Check sheet for the modelled part. Datum: model origin and axes. Units: mm. Face numbers are marked on the shaded views. A direction names the side the tool comes from. Coordinates: 2 decimals unless noted, no trailing zeros. Loops run counter-clockwise (first coordinate to the right, second up) from the corner with the lowest first, then second, coordinate; pieces in that order, holes last. Notation, with made-up numbers: (-38, -17.5) - (-12, -17.5) arc R32 cw to (-12, 13.5) - close; hole circle Ø2 at (67, 88.25). An arc over 180 degrees is marked (long way). Use a Markdown table: item, result. Add a question column.
1) Draft check along X on the marked faces 4, 5, 6 and 7. Enter one of: pulls with the +X half, pulls with the -X half, needs draft (parallel to the pull), parting line crosses it, or undercut.
2) Sectioned sample at D-D, the plane x = -8.5. Enter the section's corners in (y, z), then the cut area to 3 significant figures.
3) Sectioned sample at B-B, the plane y = -46. Enter the section's corners in (x, z), then the cut area to 3 significant figures.
4) Tool access check on the marked faces 1, 2 and 3. Record the directions out of +Z, -Z, +X, -X, +Y, -Y that give a thin tool (end or side, any length) a straight path to the whole face; none if there is none.
5) Go/stop test with flat-tipped pins: P1, Ø8, axis at y = -9, z = 138.5, coming from the +X side; P2, Ø9, axis at x = -8.5, z = 137.15, coming from the +Y side; P3, Ø2.5, axis at x = 14.5, y = -43.5, coming from the +Z side; P4, Ø6, axis at x = -1.5, z = 132.5, coming from the -Y side. Record where each tip stops, or that it passes through.
6) Sectioned sample at A-A, the plane x = 0. Enter the section's corners in (y, z).
7) Sectioned sample at C-C, the plane y = 1.5. Enter the section's corners in (x, z).
8) Thickness scan on line 1 (X direction, y = -3.2, z = 137.15); line 2 (Y direction, x = -17, z = 124); line 3 (Y direction, x = -9, z = 139). Record the ranges inside material, lowest first.
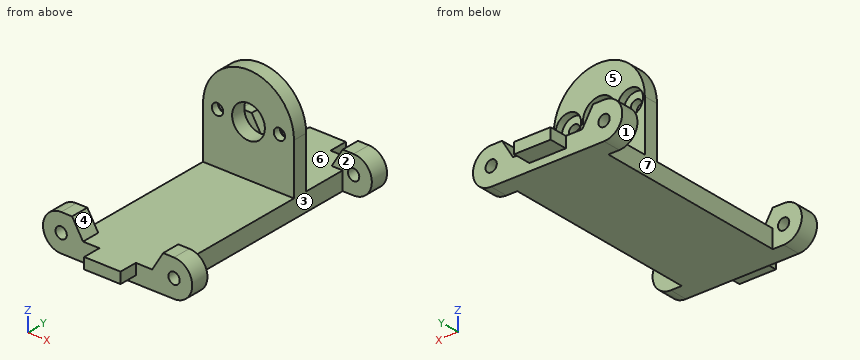
from build123d import *

# Parameters (mm, degrees)
SKETCH11_R          = 1.55
SKETCH11_R_2        = 4.5
BOSS_EXTRUDE1_DEPTH = 4
BOSS_EXTRUDE2_DEPTH = 5
SKETCH13_R          = 3.5
CUT_EXTRUDE1_DEPTH  = 2
SKETCH14_R          = 1.55
BOSS_EXTRUDE3_DEPTH = 5
BOSS_EXTRUDE4_START = -5
SKETCH15_R          = 1.55
BOSS_EXTRUDE4_DEPTH = 5
SKETCH16_W          = 10
SKETCH16_H          = 3
BOSS_EXTRUDE5_DEPTH = 5
SKETCH17_W          = 10
SKETCH17_H          = 3
BOSS_EXTRUDE6_DEPTH = 5


with BuildPart() as part:
    # Sketch11 → Boss-Extrude1 (new body)
    with BuildSketch(Plane(origin=(0, 0, 51.65), x_dir=(1, 0, 0), z_dir=(0, -1, 0))):
        with BuildLine():
            Line((12.5, 85.5), (12.5, 71.5))
            Line((12.5, 71.5), (-12.5, 71.5))
            Line((-12.5, 71.5), (-12.5, 85.5))
            ThreePointArc((-12.5, 85.5), (0, 98), (12.5, 85.5))
        make_face()
        with Locations(Location((-8.5, 85.5, 0), (0, 0, 270))):
            Circle(SKETCH11_R, mode=Mode.SUBTRACT)
        with Locations(Location((8.5, 85.5, 0), (0, 0, 270))):
            Circle(SKETCH11_R, mode=Mode.SUBTRACT)
        with Locations(Location((0, 85.5, 0), (0, 0, 270))):
            Circle(SKETCH11_R_2, mode=Mode.SUBTRACT)
    extrude(amount=BOSS_EXTRUDE1_DEPTH)

    # Sketch12 → Boss-Extrude2 (add)
    with BuildSketch(Plane(origin=(0, 0, 123.15), x_dir=(-1, 0, 0), z_dir=(0, 0, -1))):
        Polygon((-12.5, 0), (-12.5, 17), (12.5, 17), (12.5, 0), (12.5, -4), (12.5, -47), (-12.5, -47), (-12.5, -4), align=None)
    extrude(amount=BOSS_EXTRUDE2_DEPTH)

    # Sketch13 → Cut-Extrude1 (cut)
    with BuildSketch(Plane(origin=(0, 0, 0), x_dir=(1, 0, 0), z_dir=(0, 1, 0))):
        with Locations(Location((-8.5, -137.15, 0), (0, 0, 270))):
            Circle(SKETCH13_R)
        with Locations(Location((8.5, -137.15, 0), (0, 0, 270))):
            Circle(SKETCH13_R)
    extrude(amount=-CUT_EXTRUDE1_DEPTH, mode=Mode.SUBTRACT)

    # Sketch14 → Boss-Extrude3 (add)
    with BuildSketch(Plane(origin=(0, 17, 0), x_dir=(1, 0, 0), z_dir=(0, 1, 0))):
        with BuildLine():
            Line((15.5, -118.15), (-15.5, -118.15))
            ThreePointArc((-15.5, -118.15), (-20.5, -123.15), (-15.5, -128.15))
            Line((-15.5, -128.15), (-12.5, -128.15))
            Line((-12.5, -128.15), (-9.5, -123.15))
            Line((-9.5, -123.15), (9.5, -123.15))
            Line((9.5, -123.15), (12.5, -128.15))
            Line((12.5, -128.15), (15.5, -128.15))
            ThreePointArc((15.5, -128.15), (20.5, -123.15), (15.5, -118.15))
        make_face()
        with Locations(Location((-15.5, -123.15, 0), (0, 0, 270))):
            Circle(SKETCH14_R, mode=Mode.SUBTRACT)
        with Locations(Location((15.5, -123.15, 0), (0, 0, 270))):
            Circle(SKETCH14_R, mode=Mode.SUBTRACT)
    extrude(amount=-BOSS_EXTRUDE3_DEPTH)

    # Sketch15 → Boss-Extrude4 (add)
    with BuildSketch(Plane(origin=(0, -47, 0), x_dir=(-1, 0, 0), z_dir=(0, -1, 0)).offset(BOSS_EXTRUDE4_START)):
        with BuildLine():
            Line((15.5, -118.15), (-15.5, -118.15))
            ThreePointArc((-15.5, -118.15), (-20.5, -123.15), (-15.5, -128.15))
            Line((-15.5, -128.15), (-12.5, -128.15))
            Line((-12.5, -128.15), (-9.5, -123.15))
            Line((-9.5, -123.15), (9.5, -123.15))
            Line((9.5, -123.15), (12.5, -128.15))
            Line((12.5, -128.15), (15.5, -128.15))
            ThreePointArc((15.5, -128.15), (20.5, -123.15), (15.5, -118.15))
        make_face()
        with Locations(Location((15.5, -123.15, 0), (0, 0, 270))):
            Circle(SKETCH15_R, mode=Mode.SUBTRACT)
        with Locations(Location((-15.5, -123.15, 0), (0, 0, 270))):
            Circle(SKETCH15_R, mode=Mode.SUBTRACT)
    extrude(amount=BOSS_EXTRUDE4_DEPTH)

    # Sketch16 → Boss-Extrude5 (add)
    with BuildSketch(Plane.XZ.offset(47)):
        with Locations((0, 121.65)):
            Rectangle(SKETCH16_W, SKETCH16_H)
    extrude(amount=BOSS_EXTRUDE5_DEPTH)

    # Sketch17 → Boss-Extrude6 (add)
    with BuildSketch(Plane(origin=(0, 17, 0), x_dir=(1, 0, 0), z_dir=(0, 1, 0))):
        with Locations((0, -121.65)):
            Rectangle(SKETCH17_W, SKETCH17_H)
    extrude(amount=BOSS_EXTRUDE6_DEPTH)


solid = part.part
Solved:
| question | item | result |
|---|---|---|
| 1 | face 4 | undercut |
| 1 | face 5 | needs draft |
| 1 | face 6 | undercut |
| 1 | face 7 | pulls with the -X half |
| 2 | outline | (-47, 118.15) - (17, 118.15) - (17, 123.15) - (0, 123.15) - (0, 133.65) - (-2, 133.65) - (-2, 135.6) - (-4, 135.6) - (-4, 123.15) - (-47, 123.15) - close; (-4, 138.7) - (-2, 138.7) - (-2, 140.65) - (0, 140.65) - (0, 146.32) - (-4, 146.32) - close |
| 2 | area | 392 mm2 |
| 3 | outline | (-15.5, 118.15) - (15.5, 118.15) arc R5 ccw to (15.5, 128.15) - (12.5, 128.15) - (9.5, 123.15) - (-9.5, 123.15) - (-12.5, 128.15) - (-15.5, 128.15) arc R5 ccw to start; hole circle Ø3.1 at (-15.5, 123.15); hole circle Ø3.1 at (15.5, 123.15) |
| 3 | area | 263 mm2 |
| 4 | face 1 | -X, +Y, -Y |
| 4 | face 2 | +Z, +X |
| 4 | face 3 | +Z, -Z, +X |
| 5 | P1 | passes through |
| 5 | P2 | stops at y = 0 |
| 5 | P3 | stops at z = 128.15 |
| 5 | P4 | stops at y = -4 |
| 6 | outline | (-52, 120.15) - (-47, 120.15) - (-47, 118.15) - (17, 118.15) - (17, 120.15) - (22, 120.15) - (22, 123.15) - (0, 123.15) - (0, 132.65) - (-4, 132.65) - (-4, 123.15) - (-52, 123.15) - close; (-4, 141.65) - (0, 141.65) - (0, 149.65) - (-4, 149.65) - close |
| 7 | outline | (-12.5, 118.15) - (12.5, 118.15) - (12.5, 123.15) - (-12.5, 123.15) - close |
| 8 | line 1 | x = -12.5 to -10.05, -6.95 to -4.5, 4.5 to 6.95, 10.05 to 12.5 |
| 8 | line 2 | y = -47 to -42, 12 to 17 |
| 8 | line 3 | y = -4 to -2 |
